Here's how the part is built. I have some questions about the finished solid (model axes, mm). Face numbers are marked on the shaded views. Round coordinates to 2 decimals unless told otherwise and drop trailing zeros. Write each loop counter-clockwise with the first axis right and the second up, starting at its lowest first coordinate (ties: lowest second). Pieces come first, ordered by that corner, then holes. Notation, with made-up numbers: (-5, 80) -> (32, 80) arc R15 cw to (32, 108) -> close; hole circle Ø7 at (77.5, -2.5). An arc over 180 degrees is marked (long way). Answer in a Markdown table with one row per item.
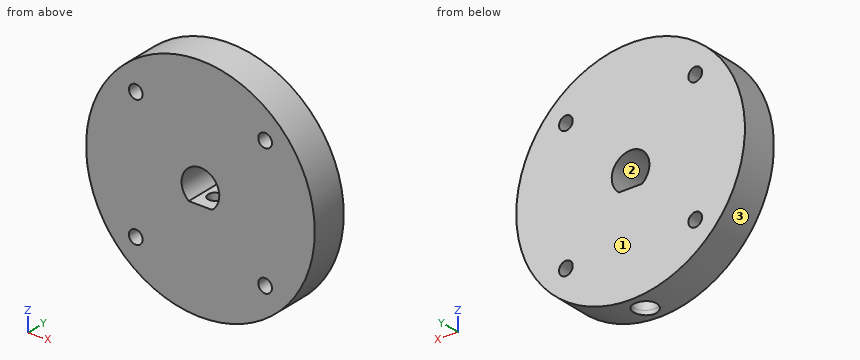
from build123d import *

# Parameters (mm, degrees)
SKETCH1_R               = 25
SKETCH1_R_2             = 1.5
BOSS_EXTRUDE1_DEPTH     = 8
SKETCH2_R               = 1.5
CUT_EXTRUDE1_DEPTH      = 35
SKETCH3_R               = 2.540300179
CUT_EXTRUDE3_DEPTH      = 2
CUT_EXTRUDE3_DEPTH_BACK = 35


with BuildPart() as part:
    # Sketch1 → Boss-Extrude1 (new body)
    with BuildSketch(Plane(origin=(0, 0, 0), x_dir=(1, 0, 0), z_dir=(0, 1, 0))):
        Circle(SKETCH1_R)
        with Locations((-14.142135624, -14.142135624)):
            Circle(SKETCH1_R_2, mode=Mode.SUBTRACT)
        with Locations((-14.142135624, 14.142135624)):
            Circle(SKETCH1_R_2, mode=Mode.SUBTRACT)
        with Locations((14.142135624, 14.142135624)):
            Circle(SKETCH1_R_2, mode=Mode.SUBTRACT)
        with Locations((14.142135624, -14.142135624)):
            Circle(SKETCH1_R_2, mode=Mode.SUBTRACT)
        with BuildLine():
            Line((2.540300179, 3.25), (-2.540300179, 3.25))
            ThreePointArc((-2.540300179, 3.25), (0, -4.125), (2.540300179, 3.25))
        make_face(mode=Mode.SUBTRACT)
    extrude(amount=BOSS_EXTRUDE1_DEPTH)

    # Sketch2 → Cut-Extrude1 (cut)
    with BuildSketch(Plane.XY.offset(-3.25)):
        with Locations((0, 4)):
            Circle(SKETCH2_R)
    extrude(amount=-CUT_EXTRUDE1_DEPTH, mode=Mode.SUBTRACT)

    # Sketch3 → Cut-Extrude3 (cut, two sides)
    with BuildSketch(Plane.XY.offset(-24)) as cut_extrude3_sk:
        with Locations((0, 4)):
            Circle(SKETCH3_R)
    extrude(amount=CUT_EXTRUDE3_DEPTH, mode=Mode.SUBTRACT)
    extrude(cut_extrude3_sk.sketch, amount=-CUT_EXTRUDE3_DEPTH_BACK, mode=Mode.SUBTRACT)


solid = part.part
1) We'd pull the mould along Z, two halves only. Please class the marked faces 1, 2 and 3: +Z half, -Z half, draft (parallel to the pull), parting line (faces both ways), or undercut.
Response:
| item | result |
|---|---|
| face 1 | draft |
| face 2 | undercut |
| face 3 | parting line |
2) For pin 1 (4 mm diameter, centred on x = 0, y = 3.5, fed in from -Z); pin 2 (2.5 mm diameter, centred on x = 14.14, z = -14.14, fed in from +Y); pin 3 (2.5 mm diameter, centred on x = 1, y = 5, fed in from +Z); pin 4 (3 mm diameter, centred on y = 3.5, z = 18.5, fed in from +X), each with a flat end and sliding along its axis, tell me the tip position at first contact or that it passes through.
Response:
| item | result |
|---|---|
| pin 1 | stops at z = -22 |
| pin 2 | passes through |
| pin 3 | stops at z = 25 |
| pin 4 | stops at x = 18.33 |
3) I want a section at B-B, the plane z = 0. List the corners of the cut face in (x, y) for me (3 decimals), and give its area (3 significant figures).
Response:
| item | result |
|---|---|
| outline | (-25, 0) -> (-4.125, 0) -> (-4.125, 8) -> (-25, 8) -> close; (4.125, 0) -> (25, 0) -> (25, 8) -> (4.125, 8) -> close |
| area | 334 mm^2 |
4) I need wall thicknesses on line 1 (Y direction, x = 0, z = -24.45); line 2 (X direction, y = 3.75, z = -15); line 3 (X direction, y = 7, z = -14). Which ranges of each line are inside material? Lowest first, please. Write a range as [from, to].
Response:
| item | result |
|---|---|
| line 1 | y = [0, 1.46], [6.54, 8] |
| line 2 | x = [-20, -15.37], [-12.91, -1.48], [1.48, 12.91], [15.37, 20] |
| line 3 | x = [-20.71, -15.64], [-12.65, 12.65], [15.64, 20.71] |
5) I want a section at C-C, the plane y = 7.25. List the corners of the cut face in (x, z) for me (3 decimals), and give its area (3 significant figures).
Response:
| item | result |
|---|---|
| outline | circle Ø50 at (0, 0); hole circle Ø3 at (-14.142, -14.142); hole circle Ø3 at (-14.142, 14.142); hole (-2.54, -3.25) -> (2.54, -3.25) arc R4.125 ccw (long way) to start; hole circle Ø3 at (14.142, -14.142); hole circle Ø3 at (14.142, 14.142) |
| area | 1,880 mm^2 |
6) I want a section at D-D, the plane y = 4. List the corners of the cut face in (x, z) for me (3 decimals).
Response:
| item | result |
|---|---|
| outline | (-2.54, -24.871) -> (-2.54, -22) -> (-1.5, -22) -> (-1.5, -3.25) -> (-2.54, -3.25) arc R4.125 cw (long way) to (2.54, -3.25) -> (1.5, -3.25) -> (1.5, -22) -> (2.54, -22) -> (2.54, -24.871) arc R25 ccw (long way) to start; hole circle Ø3 at (-14.142, -14.142); hole circle Ø3 at (-14.142, 14.142); hole circle Ø3 at (14.142, -14.142); hole circle Ø3 at (14.142, 14.142) |
7) I want a section at A-A, the plane x = 0. List the corners of the cut face in (y, z) for me (3 decimals), and give its area (3 significant figures).
Response:
| item | result |
|---|---|
| outline | (0, -25) -> (1.46, -25) -> (1.46, -22) -> (2.5, -22) -> (2.5, -3.25) -> (0, -3.25) -> close; (0, 4.125) -> (8, 4.125) -> (8, 25) -> (0, 25) -> close; (5.5, -22) -> (6.54, -22) -> (6.54, -25) -> (8, -25) -> (8, -3.25) -> (5.5, -3.25) -> close |
| area | 270 mm^2 |
